```python
from build123d import *

# Parameters (mm, degrees)
BOSS_EXTRUDE2_DEPTH = 25
SKETCH4_R           = 4
CUT_EXTRUDE1_DEPTH  = 66
SKETCH6_R           = 4
CUT_EXTRUDE2_DEPTH  = 58
CUT_EXTRUDE3_DEPTH  = 58
SKETCH9_R           = 1
CUT_EXTRUDE4_DEPTH  = 58
SKETCH10_R          = 1
CUT_EXTRUDE5_DEPTH  = 66


with BuildPart() as part:
    # Sketch3 → Boss-Extrude2 (new body)
    with BuildSketch(Plane.XY):
        Polygon((-79.925523148, 45.386502584), (-27.042967192, 45.386502584), (-24.925523148, 45.386502584), (-24.925523148, -19.613497416), (-26.925523148, -19.613497416), (-26.925523148, 43.389953837), (-79.925523148, 43.389953837), (-79.925523148, -19.613497416), (-81.925523148, -19.613497416), (-81.925523148, 45.386502584), align=None)
    extrude(amount=BOSS_EXTRUDE2_DEPTH)

    # Sketch4 → Cut-Extrude1 (cut, through all)
    with BuildSketch(Plane(origin=(0, 45.386502584, 0), x_dir=(1, 0, 0), z_dir=(0, 1, 0))):
        with Locations((-54.925523148, -12.5)):
            Circle(SKETCH4_R)
    extrude(amount=-CUT_EXTRUDE1_DEPTH, mode=Mode.SUBTRACT)

    # Sketch6 → Cut-Extrude2 (cut, through all)
    with BuildSketch(Plane.ZY.offset(81.925523148)):
        with Locations((12.5, -5.613497416)):
            Circle(SKETCH6_R)
    extrude(amount=-CUT_EXTRUDE2_DEPTH, mode=Mode.SUBTRACT)

    # Sketch8 → Cut-Extrude3 (cut, through all)
    with BuildSketch(Plane.ZY.offset(81.925523148)):
        with BuildLine():
            Line((0, -19.613497416), (12.5, -19.613497416))
            ThreePointArc((12.5, -19.613497416), (3.661165213, -15.952332159), (0, -7.113497352))
            Line((0, -7.113497352), (0, -19.613497416))
        make_face()
        with BuildLine():
            Line((12.5, -19.613497416), (25, -19.613497416))
            Line((25, -19.613497416), (25, -7.113497416))
            ThreePointArc((25, -7.113497416), (21.338834765, -15.952332181), (12.5, -19.613497416))
        make_face()
    extrude(amount=-CUT_EXTRUDE3_DEPTH, mode=Mode.SUBTRACT)

    # Sketch9 → Cut-Extrude4 (cut, through all)
    with BuildSketch(Plane(origin=(-24.925523148, 0, 0), x_dir=(0, 0, -1), z_dir=(1, 0, 0))):
        with Locations((-12.5, -11.6185898)):
            Circle(SKETCH9_R)
        with Locations((-18.505092383, -5.613497416)):
            Circle(SKETCH9_R)
        with Locations((-6.494907617, -5.613497416)):
            Circle(SKETCH9_R)
        with Locations((-12.5, 0.391594967)):
            Circle(SKETCH9_R)
    extrude(amount=-CUT_EXTRUDE4_DEPTH, mode=Mode.SUBTRACT)

    # Sketch10 → Cut-Extrude5 (cut, through all)
    with BuildSketch(Plane(origin=(0, 45.386502584, 0), x_dir=(1, 0, 0), z_dir=(0, 1, 0))):
        with Locations((-48.925524223, -12.499998866)):
            Circle(SKETCH10_R)
        with Locations((-54.925524223, -6.499998866)):
            Circle(SKETCH10_R)
        with Locations((-54.925524223, -18.499998866)):
            Circle(SKETCH10_R)
        with Locations((-60.925524223, -12.499998866)):
            Circle(SKETCH10_R)
    extrude(amount=-CUT_EXTRUDE5_DEPTH, mode=Mode.SUBTRACT)


solid = part.part
```
Check sheet for the modelled part. Datum: model origin and axes. Units: mm. A direction names the side the tool comes from. Give positions to 0.01 mm unless a question says otherwise; leave off trailing zeros. Order: outer loops, then holes, each group sorted by start corner. A loop starts at its lowest first (then second) coordinate and runs counter-clockwise, first axis right, second up. Notation, with made-up numbers: (-35.75, -23) -> (-6.75, -23) arc R8 cw to (-6.75, -10) -> close; hole circle Ø8 at (88.25, 59). An arc over 180 degrees is marked (long way). Return JSON: item names as keys, results as strings.
1. Set-up check for faces 1 (the flat face through (-79.926, 12, 12)), 2 (the cylindrical face through (-49.66, 44.4, 11.82)): record each of +Z, -Z, +X, -X, +Y, -Y from which the full face is reachable in a straight line by a thin tool's end or side.
From the geometry:
{"face 1": "+Z, -Z, -Y", "face 2": "+Y, -Y"}
2. Cross-section at C-C, the plane z = 22.75. Record the cut outline in (x, y), plus the area to 3 significant figures.
From the geometry:
{"outline": "(-81.93, -14.27) -> (-79.93, -14.27) -> (-79.93, 43.39) -> (-26.93, 43.39) -> (-26.93, -14.27) -> (-24.93, -14.27) -> (-24.93, 45.39) -> (-81.93, 45.39) -> close", "area": "344 mm^2"}
3. Cross-section at B-B, the plane y = -8.5. Record the cut outline in (x, z), plus the area to 3 significant figures.
From the geometry:
{"outline": "(-81.93, 0.08) -> (-79.93, 0.08) -> (-79.93, 9.73) -> (-81.93, 9.73) -> close; (-81.93, 15.27) -> (-79.93, 15.27) -> (-79.93, 24.92) -> (-81.93, 24.92) -> close; (-26.93, 0.08) -> (-24.93, 0.08) -> (-24.93, 9.73) -> (-26.93, 9.73) -> close; (-26.93, 15.27) -> (-24.93, 15.27) -> (-24.93, 24.92) -> (-26.93, 24.92) -> close", "area": "77.2 mm^2"}
4. Go/stop test with flat-tipped pins: P1, Ø1.6, axis at y = -5.61, z = 6.49, coming from the +X side; P2, Ø3, axis at y = -5.61, z = 6.49, coming from the -X side; P3, Ø4, axis at x = -36, z = 13.5, coming from the -Y side. Record where each tip stops, or that it passes through.
From the geometry:
{"P1": "through", "P2": "x = -81.93", "P3": "y = 43.39"}
5. Mould release check, pull along X, two halves, no side actions. Record for faces 3 (the flat face through (-81.926, 12, 12)), 4 (the cylindrical face through (-25.912, -10.943, 13.237)), 5 (the cylindrical face through (-59.97, 44.4, 12.2)): +X half, -X half, draft (parallel to the pull), parting line (faces both ways), or undercut.
From the geometry:
{"face 3": "-X half", "face 4": "draft", "face 5": "undercut"}
6. Cross-section at D-D, the plane x = -71.5. Record the cut outline in (y, z).
From the geometry:
{"outline": "(43.39, 0) -> (45.39, 0) -> (45.39, 25) -> (43.39, 25) -> close"}
7. Cross-section at A-A, the plane y = 3.5. Record the cut outline in (x, z), plus the area to 3 significant figures.
From the geometry:
{"outline": "(-81.93, 0) -> (-79.93, 0) -> (-79.93, 25) -> (-81.93, 25) -> close; (-26.93, 0) -> (-24.93, 0) -> (-24.93, 25) -> (-26.93, 25) -> close", "area": "100 mm^2"}
8. Material ranges on probe 1 along Y at (x, z) = (-26.25, 12.5); probe 2 along X at (y, z) = (27, 9.5); probe 3 along Y at (x, z) = (-72.5, 12.25), recorded low to high. Write a range as [from, to].
From the geometry:
{"probe 1": "[-19.61, -12.62], [-10.62, -9.61], [-1.61, -0.61], [1.39, 45.39]", "probe 2": "[-81.93, -79.93], [-26.93, -24.93]", "probe 3": "[43.39, 45.39]"}
